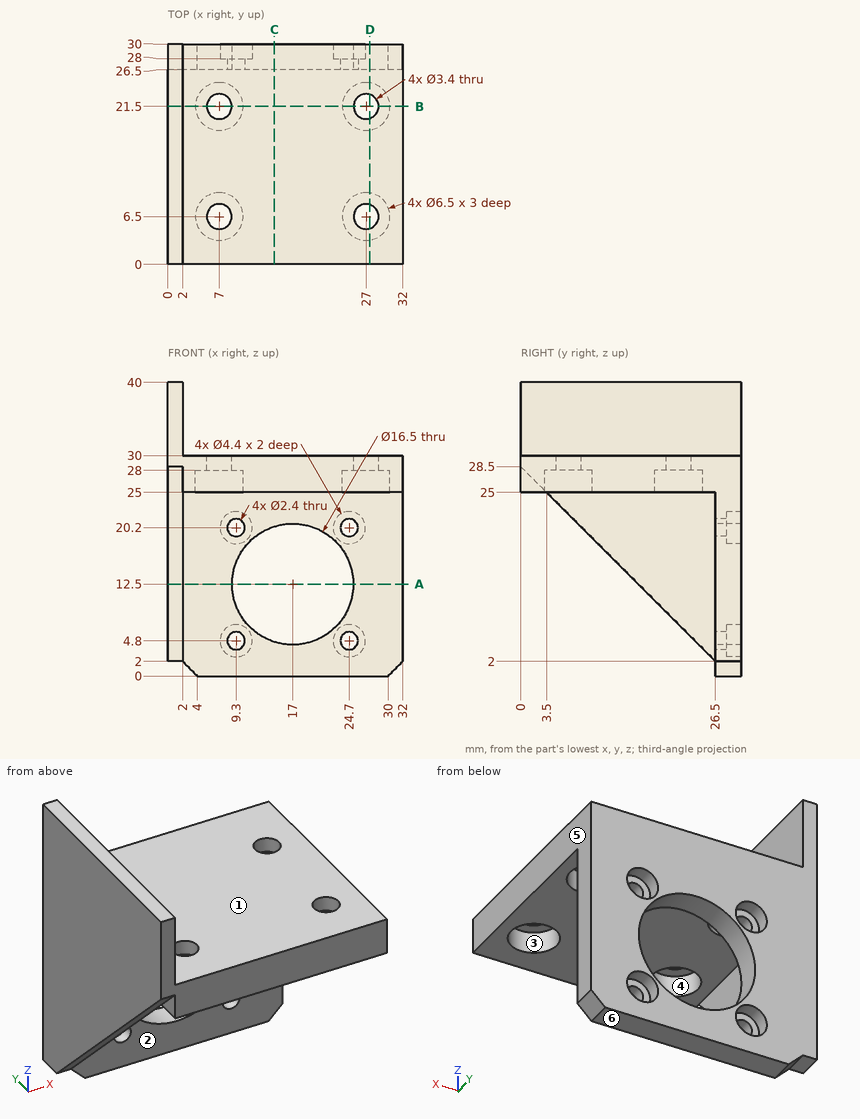
Source: three-view drawing plus pictorial views. Frame: mm from the lowest corner of the part. A direction names the side the tool comes from. Coordinates: 2 decimals unless noted, no trailing zeros. Write each loop counter-clockwise with the first axis right and the second up, starting at its lowest first coordinate (ties: lowest second). Pieces come first, ordered by that corner, then holes. Notation, with made-up numbers: (5.25, -9) - (39.25, -9) arc R21 ccw to (39.25, 22) - close; hole circle Ø3 at (-23.5, -14). An arc over 180 degrees is marked (long way). Return JSON: item names as keys, results as strings.
Item 1: Pull-direction query (X, two-part tool) for the marked faces 4, 5 and 6; classes: +X half, -X half, draft (parallel to the pull), parting line (faces both ways), or undercut.
Completed:
{"face 4": "undercut", "face 5": "+X half", "face 6": "draft"}
Item 2: Section query D-D (x = 27.5). Output: boundary loops of the cut face in (y, z).
Completed:
{"outline": "(0, 25) - (3.29, 25) - (3.29, 28) - (4.88, 28) - (4.88, 30) - (0, 30) - close; (8.12, 28) - (9.71, 28) - (9.71, 25) - (18.29, 25) - (18.29, 28) - (19.88, 28) - (19.88, 30) - (8.12, 30) - close; (23.12, 28) - (24.71, 28) - (24.71, 25) - (26.5, 25) - (26.5, 0) - (30, 0) - (30, 30) - (23.12, 30) - close"}
Item 3: Pin query (flat end, axial travel): pin 1 Ø3 at (x, y) = (27.5, 22) entering from -Z; pin 2 Ø5 at (y, z) = (21, 36) entering from +X; pin 3 Ø2 at (x, y) = (6, 19.5) entering from +Z. Return the tip coordinate at first contact, or that it passes through.
Completed:
{"pin 1": "stops at z = 28", "pin 2": "stops at x = 2", "pin 3": "stops at z = 30"}
Item 4: Section query C-C (x = 14.5). Output: boundary loops of the cut face in (y, z).
Completed:
{"outline": "(0, 25) - (26.5, 25) - (26.5, 20.36) - (30, 20.36) - (30, 30) - (0, 30) - close; (26.5, 0) - (30, 0) - (30, 4.64) - (26.5, 4.64) - close"}
Item 5: Section query A-A (z = 12.5). Output: boundary loops of the cut face in (x, y), and give its area (4 significant figures).
Completed:
{"outline": "(0, 16) - (2, 16) - (2, 26.5) - (8.75, 26.5) - (8.75, 30) - (0, 30) - close; (25.25, 26.5) - (32, 26.5) - (32, 30) - (25.25, 30) - close", "area": "75.25 mm2"}
Item 6: Line query: L1, parallel to X at y = 21.5, z = 27.35; L2, parallel to Y at x = 7, z = 26; L3, parallel to X at y = 25.75, z = 10. Output: solid intervals per line, ascending.
Completed:
{"L1": "x = 0 to 3.75, 10.25 to 23.75, 30.25 to 32", "L2": "y = 0 to 3.25, 9.75 to 18.25, 24.75 to 30", "L3": "x = 0 to 2"}
Item 7: Section query B-B (y = 21.5). Output: boundary loops of the cut face in (x, z), and give its area (3 significant figures).
Completed:
{"outline": "(0, 7) - (2, 7) - (2, 25) - (3.75, 25) - (3.75, 28) - (5.3, 28) - (5.3, 30) - (2, 30) - (2, 40) - (0, 40) - close; (8.7, 28) - (10.25, 28) - (10.25, 25) - (23.75, 25) - (23.75, 28) - (25.3, 28) - (25.3, 30) - (8.7, 30) - close; (28.7, 28) - (30.25, 28) - (30.25, 25) - (32, 25) - (32, 30) - (28.7, 30) - close", "area": "163 mm2"}
Item 8: Reachability of the marked faces 1, 2 and 3 from +Z, -Z, +X, -X, +Y, -Y: full face, straight path, thin tool, end or side. Return the list, or none.
Completed:
{"face 1": "+Z, +X, +Y, -Y", "face 2": "-Z, +X, -Y", "face 3": "-Z"}
